Model file for the job. Use its own axes, mm. Face numbers are marked on the shaded views. Round coordinates to 2 decimals unless told otherwise and drop trailing zeros. Loops run counter-clockwise (first coordinate to the right, second up) from the corner with the lowest first, then second, coordinate; pieces in that order, holes last. Notation, with made-up numbers: M 84.5,15.25 L 117.5,15.25 A21 cw 117.5,34.25 Z; hole C 40,24.25 d4. An arc over 180 degrees is marked long. Use a Markdown table: item, result. Add a question column.
Item 1: Saw through at C-C on z = 3.75. Write the cut outline in (x, y) (3 decimals).
Item 2: Saw through at D-D on x = 2. Write the cut outline in (y, z).
Item 3: Two-plate mould, pull along X, no slides. Class the marked faces 1, 2 and 3: +X half, -X half, draft (parallel to the pull), parting line (faces both ways), or undercut.
Item 4: Pin check, flat tip, straight feed: P1, Ø2, axis at y = -1.5, z = 3.5, coming from the +X side. Stop position of the tip, or through.
Item 5: Saw through at A-A on y = 0. Write the cut outline in (x, z) (3 decimals), then the cut area to 3 significant figures.
Item 6: Wall check: L1, parallel to Y at x = 0, z = 3.05 (3 decimals); L2, parallel to Z at x = 0, y = 1; L3, parallel to Y at x = -1, z = 0.5. Give the ranges that are in metal, low to high. Write a range as from..to.
```python
from build123d import *

# Parameters (mm, degrees)
F0_R     = 3.1496
F0_R_2   = 1.905
F1_DEPTH = 1.778
F2_DEPTH = 6.35
F3_R     = 3.070911
F4_DEPTH = 1.25


with BuildPart() as f1:
    # F0 (on Top) → F1 (new body)
    with BuildSketch(Plane.XY):
        Circle(F0_R)
        Circle(F0_R_2, mode=Mode.SUBTRACT)
    extrude(amount=F1_DEPTH)

    # F0 (on Top) → F2 (join)
    with BuildSketch(Plane.XY):
        Circle(F0_R)
        Circle(F0_R_2, mode=Mode.SUBTRACT)
    extrude(amount=F2_DEPTH)

    # F3 (on face) → F4 (join)
    with BuildSketch(Plane.XY.offset(6.35)):
        Circle(F3_R)
    extrude(amount=-F4_DEPTH)


solid = f1.part
```
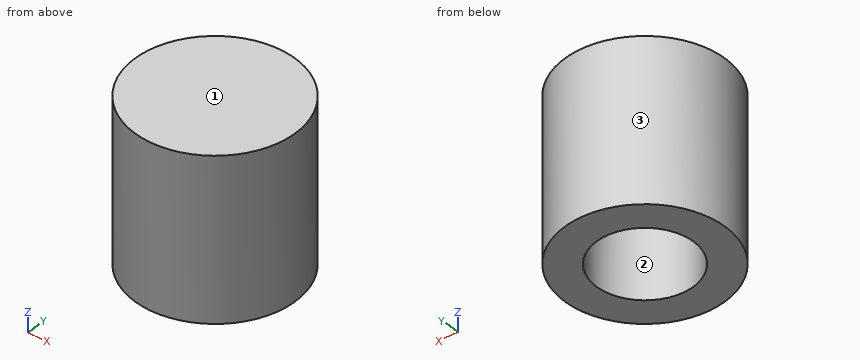
Entries:
| question | item | result |
|---|---|---|
| 1 | outline | C 0,0 d6.299; hole C 0,0 d3.81 |
| 2 | outline | M -2.43,0 L 2.43,0 L 2.43,6.35 L -2.43,6.35 Z |
| 3 | face 1 | draft |
| 3 | face 2 | undercut |
| 3 | face 3 | parting line |
| 4 | P1 | x = 3.11 |
| 5 | outline | M -3.15,0 L -1.905,0 L -1.905,5.1 L 1.905,5.1 L 1.905,0 L 3.15,0 L 3.15,6.35 L -3.15,6.35 Z |
| 5 | area | 20.6 mm2 |
| 6 | L1 | -3.15..-1.905, 1.905..3.15 |
| 6 | L2 | 5.1..6.35 |
| 6 | L3 | -2.99..-1.62, 1.62..2.99 |
